Drawing for the job (mm, zero at the part's lowest x, y, z). Coordinates: 2 decimals unless noted, no trailing zeros. Loops run counter-clockwise (first coordinate to the right, second up) from the corner with the lowest first, then second, coordinate; pieces in that order, holes last. Notation, with made-up numbers: (41.25, 55) - (70.25, 55) arc R19 cw to (70.25, 92) - close; hole circle Ø7 at (58, -27). An arc over 180 degrees is marked (long way). Put each result on its own line as item: value.
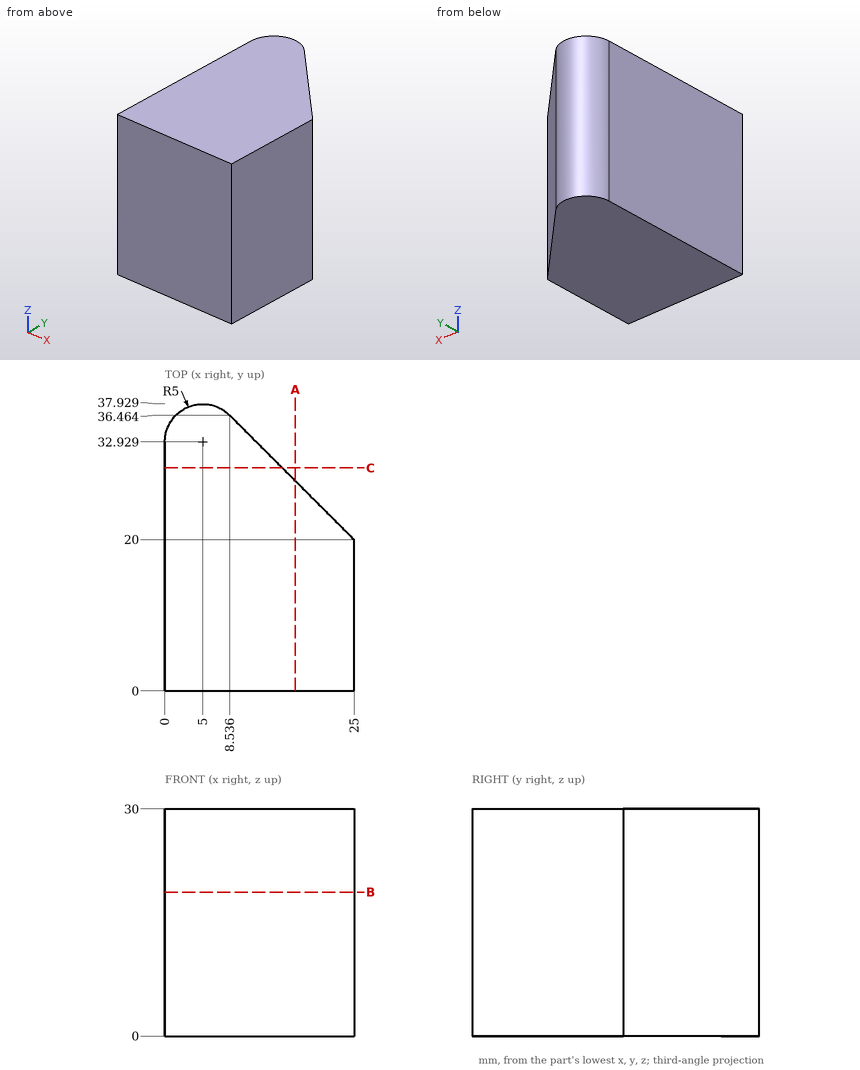
Q1. Wall check: L1, parallel to Y at x = 15, z = 26.5; L2, parallel to Y at x = 12.75, z = 15; L3, parallel to X at y = 27.5, z = 22. Give the ranges that are in metal, low to high. Write a range as from..to.
Determined:
L1: 0..30
L2: 0..32.25
L3: 0..17.5
Q2. Slice it at C-C, the plane y = 29.5. Give the cut face in (x, z).
Determined:
outline: (0, 0) - (15.5, 0) - (15.5, 30) - (0, 30) - close
Q3. Slice it at A-A, the plane x = 17.25. Give the cut face in (y, z).
Determined:
outline: (0, 0) - (27.75, 0) - (27.75, 30) - (0, 30) - close
Q4. Pin check, flat tips, straight feed: pin 1 Ø6 at (y, z) = (33.5, 5.5) entering from +X; pin 2 Ø1.5 at (x, z) = (2.5, 23) entering from +Y. Stop position of each tip, or through.
Determined:
pin 1: x = 14.5
pin 2: y = 37.61
Q5. Slice it at B-B, the plane z = 19. Give the cut face in (x, y) (1 decimal).
Determined:
outline: (0, 0) - (25, 0) - (25, 20) - (8.5, 36.5) arc R5 ccw to (0, 32.9) - close
